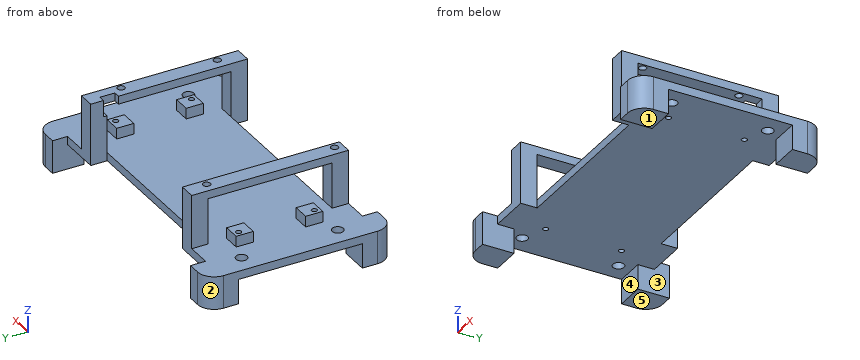
```python
from build123d import *

# Parameters (mm, degrees)
SKETCH1_W             = 112.9284
SKETCH1_H             = 57.214943904
BOSS_EXTRUDE1_DEPTH   = 3.81
BOSS_EXTRUDE2_START   = 11.43
BOSS_EXTRUDE2_DEPTH   = 11.43
CUT_EXTRUDE1_REACH    = 85.521
SKETCH3_R             = 2.58
SKETCH4_W             = 7.786771744
SKETCH4_H             = 7.895685894
BOSS_EXTRUDE3_DEPTH   = 5
CUT_EXTRUDE2_REACH    = 86.577
SKETCH5_R             = 1.25
SKETCH8_W             = 7.62
SKETCH8_H             = 7.62
BOSS_EXTRUDE4_DEPTH   = 24.892
BOSS_EXTRUDE4_2_DEPTH = 24.892
BOSS_EXTRUDE4_3_DEPTH = 24.892
BOSS_EXTRUDE4_4_DEPTH = 24.892
SKETCH9_W             = 7.62
SKETCH9_H             = 7.62
BOSS_EXTRUDE5_DEPTH   = 3.81
BOSS_EXTRUDE6_REACH   = 106.193
SKETCH10_W            = 7.62
SKETCH10_H            = 3.70730408
BOSS_EXTRUDE7_REACH   = 128.11
SKETCH11_W            = 3.81
SKETCH11_H            = 7.62
BOSS_EXTRUDE8_REACH   = 128.11
SKETCH12_W            = 3.81
SKETCH12_H            = 7.62
SKETCH14_R            = 1.7018
CUT_EXTRUDE3_DEPTH    = 3.81
SKETCH16_W            = 2.93944059
SKETCH16_H            = 6.893445181
CUT_EXTRUDE4_DEPTH    = 7.62


with BuildPart() as part:
    # Sketch1 → Boss-Extrude1 (new body)
    with BuildSketch(Plane.XY):
        with BuildLine():
            Line((-56.4642, -28.607471952), (-56.4642, 28.607471952))
            Line((-56.4642, 28.607471952), (-56.4642, 43.18))
            Line((-56.4642, 43.18), (-62.23, 43.18))
            ThreePointArc((-62.23, 43.18), (-67.618153673, 40.948153673), (-69.85, 35.56))
            Line((-69.85, 35.56), (-69.85, -35.56))
            ThreePointArc((-69.85, -35.56), (-67.618153673, -40.948153673), (-62.23, -43.18))
            Line((-62.23, -43.18), (-56.4642, -43.18))
            Line((-56.4642, -43.18), (-56.4642, -28.607471952))
        make_face()
        Rectangle(SKETCH1_W, SKETCH1_H)
        with BuildLine():
            Line((56.4642, 43.18), (56.4642, 28.607471952))
            Line((56.4642, 28.607471952), (56.4642, -28.607471952))
            Line((56.4642, -28.607471952), (56.4642, -43.18))
            Line((56.4642, -43.18), (62.23, -43.18))
            ThreePointArc((62.23, -43.18), (67.618153673, -40.948153673), (69.85, -35.56))
            Line((69.85, -35.56), (69.85, 35.56))
            ThreePointArc((69.85, 35.56), (67.618153673, 40.948153673), (62.23, 43.18))
            Line((62.23, 43.18), (56.4642, 43.18))
        make_face()
    extrude(amount=BOSS_EXTRUDE1_DEPTH)

    # Sketch2 → Boss-Extrude2 (add)
    with BuildSketch(Plane(origin=(0, 0, 0), x_dir=(-1, 0, 0), z_dir=(0, 0, -1)).offset(BOSS_EXTRUDE2_START)):
        with BuildLine():
            Line((-62.23, 43.18), (-56.4642, 43.18))
            Line((-56.4642, 43.18), (-56.4642, 28.607471952))
            Line((-56.4642, 28.607471952), (-69.85, 28.607471952))
            Line((-69.85, 28.607471952), (-69.85, 35.56))
            ThreePointArc((-69.85, 35.56), (-67.618153673, 40.948153673), (-62.23, 43.18))
        make_face()
        with BuildLine():
            Line((69.85, 28.607471952), (56.4642, 28.607471952))
            Line((56.4642, 28.607471952), (56.4642, 43.18))
            Line((56.4642, 43.18), (62.23, 43.18))
            ThreePointArc((62.23, 43.18), (67.618153673, 40.948153673), (69.85, 35.56))
            Line((69.85, 35.56), (69.85, 28.607471952))
        make_face()
        with BuildLine():
            Line((69.85, -35.56), (69.85, -28.607471952))
            Line((69.85, -28.607471952), (56.4642, -28.607471952))
            Line((56.4642, -28.607471952), (56.4642, -43.18))
            Line((56.4642, -43.18), (62.23, -43.18))
            ThreePointArc((62.23, -43.18), (67.618153673, -40.948153673), (69.85, -35.56))
        make_face()
        with BuildLine():
            Line((-69.85, -28.607471952), (-56.4642, -28.607471952))
            Line((-56.4642, -28.607471952), (-56.4642, -43.18))
            Line((-56.4642, -43.18), (-62.23, -43.18))
            ThreePointArc((-62.23, -43.18), (-67.618153673, -40.948153673), (-69.85, -35.56))
            Line((-69.85, -35.56), (-69.85, -28.607471952))
        make_face()
    extrude(amount=-BOSS_EXTRUDE2_DEPTH)

    # Sketch3 → Cut-Extrude1 (cut, up to next)
    with BuildSketch(Plane.XY.offset(3.81), mode=Mode.PRIVATE) as cut_extrude1_sk1:
        with Locations((-61.0842, 22.2292)):
            Circle(SKETCH3_R)
    cut_extrude1_tool1 = extrude(cut_extrude1_sk1.sketch, amount=-CUT_EXTRUDE1_REACH, mode=Mode.PRIVATE) & part.part
    # Sketch3 → Cut-Extrude1 (cut, up to next)
    with BuildSketch(Plane.XY.offset(3.81), mode=Mode.PRIVATE) as cut_extrude1_sk2:
        with Locations((-61.0842, -22.2208)):
            Circle(SKETCH3_R)
    cut_extrude1_tool2 = extrude(cut_extrude1_sk2.sketch, amount=-CUT_EXTRUDE1_REACH, mode=Mode.PRIVATE) & part.part
    # Sketch3 → Cut-Extrude1 (cut, up to next)
    with BuildSketch(Plane.XY.offset(3.81), mode=Mode.PRIVATE) as cut_extrude1_sk3:
        with Locations((61.0958, -22.2208)):
            Circle(SKETCH3_R)
    cut_extrude1_tool3 = extrude(cut_extrude1_sk3.sketch, amount=-CUT_EXTRUDE1_REACH, mode=Mode.PRIVATE) & part.part
    # Sketch3 → Cut-Extrude1 (cut, up to next)
    with BuildSketch(Plane.XY.offset(3.81), mode=Mode.PRIVATE) as cut_extrude1_sk4:
        with Locations((61.0958, 22.2292)):
            Circle(SKETCH3_R)
    cut_extrude1_tool4 = extrude(cut_extrude1_sk4.sketch, amount=-CUT_EXTRUDE1_REACH, mode=Mode.PRIVATE) & part.part
    add(cut_extrude1_tool1.solids().sort_by_distance((-61.0842, 22.2292, 3.81))[0], mode=Mode.SUBTRACT)
    add(cut_extrude1_tool2.solids().sort_by_distance((-61.0842, -22.2208, 3.81))[0], mode=Mode.SUBTRACT)
    add(cut_extrude1_tool3.solids().sort_by_distance((61.0958, -22.2208, 3.81))[0], mode=Mode.SUBTRACT)
    add(cut_extrude1_tool4.solids().sort_by_distance((61.0958, 22.2292, 3.81))[0], mode=Mode.SUBTRACT)

    # Sketch4 → Boss-Extrude3 (add)
    with BuildSketch(Plane.XY.offset(3.81)):
        with Locations((-48.862414128, 16.054657053)):
            Rectangle(SKETCH4_W, SKETCH4_H)
        with Locations((48.862414128, 16.054657053)):
            Rectangle(SKETCH4_W, SKETCH4_H)
        with Locations((48.862414128, -16.054657053)):
            Rectangle(SKETCH4_W, SKETCH4_H)
        with Locations((-48.862414128, -16.054657053)):
            Rectangle(SKETCH4_W, SKETCH4_H)
    extrude(amount=BOSS_EXTRUDE3_DEPTH)

    # Sketch5 → Cut-Extrude2 (cut, up to next)
    with BuildSketch(Plane.XY.offset(8.81), mode=Mode.PRIVATE) as cut_extrude2_sk1:
        with Locations((50.2442, 17.5025)):
            Circle(SKETCH5_R)
    cut_extrude2_tool1 = extrude(cut_extrude2_sk1.sketch, amount=-CUT_EXTRUDE2_REACH, mode=Mode.PRIVATE) & part.part
    # Sketch5 → Cut-Extrude2 (cut, up to next)
    with BuildSketch(Plane.XY.offset(8.81), mode=Mode.PRIVATE) as cut_extrude2_sk2:
        with Locations((50.2442, -17.4975)):
            Circle(SKETCH5_R)
    cut_extrude2_tool2 = extrude(cut_extrude2_sk2.sketch, amount=-CUT_EXTRUDE2_REACH, mode=Mode.PRIVATE) & part.part
    # Sketch5 → Cut-Extrude2 (cut, up to next)
    with BuildSketch(Plane.XY.offset(8.81), mode=Mode.PRIVATE) as cut_extrude2_sk3:
        with Locations((-50.2558, -17.4975)):
            Circle(SKETCH5_R)
    cut_extrude2_tool3 = extrude(cut_extrude2_sk3.sketch, amount=-CUT_EXTRUDE2_REACH, mode=Mode.PRIVATE) & part.part
    # Sketch5 → Cut-Extrude2 (cut, up to next)
    with BuildSketch(Plane.XY.offset(8.81), mode=Mode.PRIVATE) as cut_extrude2_sk4:
        with Locations((-50.2558, 17.5025)):
            Circle(SKETCH5_R)
    cut_extrude2_tool4 = extrude(cut_extrude2_sk4.sketch, amount=-CUT_EXTRUDE2_REACH, mode=Mode.PRIVATE) & part.part
    add(cut_extrude2_tool1.solids().sort_by_distance((50.2442, 17.5025, 8.81))[0], mode=Mode.SUBTRACT)
    add(cut_extrude2_tool2.solids().sort_by_distance((50.2442, -17.4975, 8.81))[0], mode=Mode.SUBTRACT)
    add(cut_extrude2_tool3.solids().sort_by_distance((-50.2558, -17.4975, 8.81))[0], mode=Mode.SUBTRACT)
    add(cut_extrude2_tool4.solids().sort_by_distance((-50.2558, 17.5025, 8.81))[0], mode=Mode.SUBTRACT)



with BuildPart() as body_2:
    # Sketch8 → Boss-Extrude4 (new body)
    with BuildSketch(Plane.XY.offset(3.81)):
        with Locations((-41.297898441, 32.417471952)):
            Rectangle(SKETCH8_W, SKETCH8_H)
    extrude(amount=BOSS_EXTRUDE4_DEPTH)


with BuildPart() as body_3:
    # Sketch8 → Boss-Extrude4 2 (new body)
    with BuildSketch(Plane.XY.offset(3.81)):
        with Locations((41.297898441, 32.417471952)):
            Rectangle(SKETCH8_W, SKETCH8_H)
    extrude(amount=BOSS_EXTRUDE4_2_DEPTH)


with BuildPart() as body_4:
    # Sketch8 → Boss-Extrude4 3 (new body)
    with BuildSketch(Plane.XY.offset(3.81)):
        with Locations((41.297898441, -32.417471952)):
            Rectangle(SKETCH8_W, SKETCH8_H)
    extrude(amount=BOSS_EXTRUDE4_3_DEPTH)


with BuildPart() as body_5:
    # Sketch8 → Boss-Extrude4 4 (new body)
    with BuildSketch(Plane.XY.offset(3.81)):
        with Locations((-41.297898441, -32.417471952)):
            Rectangle(SKETCH8_W, SKETCH8_H)
    extrude(amount=BOSS_EXTRUDE4_4_DEPTH)


with BuildPart() as part_1:
    add(part.part)

    add(body_2.part)  # Boss-Extrude5 merges body 2

    add(body_3.part)  # Boss-Extrude5 merges body 3

    add(body_4.part)  # Boss-Extrude5 merges body 4

    add(body_5.part)  # Boss-Extrude5 merges body 5
    # Sketch9 → Boss-Extrude5 (add)
    with BuildSketch(Plane.XY.offset(3.81)):
        with Locations((41.297898441, 32.417471952)):
            Rectangle(SKETCH9_W, SKETCH9_H)
        with Locations((-41.297898441, 32.417471952)):
            Rectangle(SKETCH9_W, SKETCH9_H)
        with Locations((-41.297898441, -32.417471952)):
            Rectangle(SKETCH9_W, SKETCH9_H)
        with Locations((41.297898441, -32.417471952)):
            Rectangle(SKETCH9_W, SKETCH9_H)
    extrude(amount=-BOSS_EXTRUDE5_DEPTH)

    # Sketch10 → Boss-Extrude6 (add, up to next)
    with BuildSketch(Plane(origin=(0, -28.607471952, 0), x_dir=(1, 0, 0), z_dir=(0, 1, 0)), mode=Mode.PRIVATE) as boss_extrude6_sk1:
        with Locations((-41.297898441, -26.84834796)):
            Rectangle(SKETCH10_W, SKETCH10_H)
    boss_extrude6_tool1 = extrude(boss_extrude6_sk1.sketch, amount=BOSS_EXTRUDE6_REACH, mode=Mode.PRIVATE) - part_1.part
    # Sketch10 → Boss-Extrude6 (add, up to next)
    with BuildSketch(Plane(origin=(0, -28.607471952, 0), x_dir=(1, 0, 0), z_dir=(0, 1, 0)), mode=Mode.PRIVATE) as boss_extrude6_sk2:
        with Locations((41.297898441, -26.84834796)):
            Rectangle(SKETCH10_W, SKETCH10_H)
    boss_extrude6_tool2 = extrude(boss_extrude6_sk2.sketch, amount=BOSS_EXTRUDE6_REACH, mode=Mode.PRIVATE) - part_1.part
    add(boss_extrude6_tool1.solids().sort_by_distance((-41.297898, -28.607472, 26.848348))[0])
    add(boss_extrude6_tool2.solids().sort_by_distance((41.297898, -28.607472, 26.848348))[0])

    # Sketch11 → Boss-Extrude7 (add, up to next)
    with BuildSketch(Plane.ZY.offset(45.107898441), mode=Mode.PRIVATE) as boss_extrude7_sk1:
        with Locations((1.905, -32.417471952)):
            Rectangle(SKETCH11_W, SKETCH11_H)
    boss_extrude7_tool1 = extrude(boss_extrude7_sk1.sketch, amount=BOSS_EXTRUDE7_REACH, mode=Mode.PRIVATE) - part_1.part
    # Sketch11 → Boss-Extrude7 (add, up to next)
    with BuildSketch(Plane.ZY.offset(45.107898441), mode=Mode.PRIVATE) as boss_extrude7_sk2:
        with Locations((1.905, 32.417471952)):
            Rectangle(SKETCH11_W, SKETCH11_H)
    boss_extrude7_tool2 = extrude(boss_extrude7_sk2.sketch, amount=BOSS_EXTRUDE7_REACH, mode=Mode.PRIVATE) - part_1.part
    add(boss_extrude7_tool1.solids().sort_by_distance((-45.107898, -32.417472, 1.905))[0])
    add(boss_extrude7_tool2.solids().sort_by_distance((-45.107898, 32.417472, 1.905))[0])

    # Sketch12 → Boss-Extrude8 (add, up to next)
    with BuildSketch(Plane(origin=(45.107898441, 0, 0), x_dir=(0, 0, -1), z_dir=(1, 0, 0)), mode=Mode.PRIVATE) as boss_extrude8_sk1:
        with Locations((-1.905, 32.417471952)):
            Rectangle(SKETCH12_W, SKETCH12_H)
    boss_extrude8_tool1 = extrude(boss_extrude8_sk1.sketch, amount=BOSS_EXTRUDE8_REACH, mode=Mode.PRIVATE) - part_1.part
    # Sketch12 → Boss-Extrude8 (add, up to next)
    with BuildSketch(Plane(origin=(45.107898441, 0, 0), x_dir=(0, 0, -1), z_dir=(1, 0, 0)), mode=Mode.PRIVATE) as boss_extrude8_sk2:
        with Locations((-1.905, -32.417471952)):
            Rectangle(SKETCH12_W, SKETCH12_H)
    boss_extrude8_tool2 = extrude(boss_extrude8_sk2.sketch, amount=BOSS_EXTRUDE8_REACH, mode=Mode.PRIVATE) - part_1.part
    add(boss_extrude8_tool1.solids().sort_by_distance((45.107898, 32.417472, 1.905))[0])
    add(boss_extrude8_tool2.solids().sort_by_distance((45.107898, -32.417472, 1.905))[0])

    # Sketch14 → Cut-Extrude3 (cut)
    with BuildSketch(Plane.XY.offset(28.702)):
        with Locations((-40.34905784, 26.641762983)):
            Circle(SKETCH14_R)
        with Locations((-40.34905784, -32.445162443)):
            Circle(SKETCH14_R)
        with Locations((42.691835463, 19.276786892)):
            Circle(SKETCH14_R)
        with Locations((42.691835463, -25.172251079)):
            Circle(SKETCH14_R)
    extrude(amount=-CUT_EXTRUDE3_DEPTH, mode=Mode.SUBTRACT)

    # Sketch16 → Cut-Extrude4 (cut)
    with BuildSketch(Plane.XY.offset(28.702)):
        with Locations((38.957618736, 26.875922591)):
            Rectangle(SKETCH16_W, SKETCH16_H)
    extrude(amount=-CUT_EXTRUDE4_DEPTH, mode=Mode.SUBTRACT)


solid = part_1.part
```
Model file for the job. Use its own axes, mm. Face numbers are marked on the shaded views. A direction names the side the tool comes from. Coordinates: 2 decimals unless noted, no trailing zeros. Order: outer loops, then holes, each group sorted by start corner. A loop starts at its lowest first (then second) coordinate and runs counter-clockwise, first axis right, second up. Notation, with made-up numbers: (69, 58.25) - (123, 58.25) arc R12 ccw to (123, 72.25) - close; hole circle Ø3 at (35.5, -39.5). An arc over 180 degrees is marked (long way). Return JSON: item names as keys, results as strings. Group by question number.
1) Mould opens along X. For the marked faces 1, 2 and 3 say: released by +X, released by -X, zero draft, split by the parting line, or undercut.
2) Saw through at A-A, the plane y = -9.5. Write the cut outline in (x, z).
3) Probe line 1 (Y direction, x = 57, z = -8.5); line 2 (Z direction, x = -26, y = -16.5); line 3 (Z direction, x = -61, y = -38.5). List the from-to ranges inside material, lowest first. Write a range as from..to.
4) Flat gauge pins, fed straight in: P1, Ø5.5, axis at x = -43, z = 9, coming from the -Y side; P2, Ø2.5, axis at x = -40, z = 18.5, coming from the +Y side; P3, Ø1.5, axis at x = 50, z = 5.5, coming from the -Y side; P4, Ø12, axis at y = 33, z = 5.5, coming from the +X side. Where does each tip first touch, or does it go through?
5) Saw through at C-C, the plane x = 47. Write the cut outline in (y, z).
6) Saw through at D-D, the plane z = 14.5. Write the cut outline in (x, y).
7) Tool access for the marked faces 4 and 5: list every direction of +Z, -Z, +X, -X, +Y, -Y with a clear straight run to the whole face (end or side of a thin tool).
8) Saw through at B-B, the plane z = -9. Write the cut outline in (x, y), plus the area to 3 significant figures.
Values found:
{
 "1": {"face 1": "zero draft", "face 2": "released by -X", "face 3": "undercut"},
 "2": {"outline": "(-69.85, 0) - (69.85, 0) - (69.85, 3.81) - (-69.85, 3.81) - close; (-45.11, 24.99) - (-37.49, 24.99) - (-37.49, 28.7) - (-45.11, 28.7) - close; (37.49, 24.99) - (45.11, 24.99) - (45.11, 28.7) - (37.49, 28.7) - close"},
 "3": {"line 1": "y = -43.18..-28.61, 28.61..43.18", "line 2": "z = 0..3.81", "line 3": "z = -11.43..3.81"},
 "4": {"P1": "stops at y = -36.23", "P2": "stops at y = 36.23", "P3": "stops at y = -20", "P4": "stops at x = 69.85"},
 "5": {"outline": "(-36.23, 0) - (36.23, 0) - (36.23, 3.81) - (20, 3.81) - (20, 8.81) - (12.11, 8.81) - (12.11, 3.81) - (-12.11, 3.81) - (-12.11, 8.81) - (-20, 8.81) - (-20, 3.81) - (-36.23, 3.81) - close"},
 "6": {"outline": "(-45.11, -36.23) - (-37.49, -36.23) - (-37.49, -28.61) - (-45.11, -28.61) - close; (-45.11, 28.61) - (-37.49, 28.61) - (-37.49, 36.23) - (-45.11, 36.23) - close; (37.49, -36.23) - (45.11, -36.23) - (45.11, -28.61) - (37.49, -28.61) - close; (37.49, 28.61) - (45.11, 28.61) - (45.11, 36.23) - (37.49, 36.23) - close"},
 "7": {"face 4": "-Z, +X, -X", "face 5": "-Z, +X, -X, +Y, -Y"},
 "8": {"outline": "(-69.85, -35.56) arc R7.62 ccw to (-62.23, -43.18) - (-56.46, -43.18) - (-56.46, -28.61) - (-69.85, -28.61) - close; (-69.85, 28.61) - (-56.46, 28.61) - (-56.46, 43.18) - (-62.23, 43.18) arc R7.62 ccw to (-69.85, 35.56) - close; (56.46, -43.18) - (62.23, -43.18) arc R7.62 ccw to (69.85, -35.56) - (69.85, -28.61) - (56.46, -28.61) - close; (56.46, 28.61) - (69.85, 28.61) - (69.85, 35.56) arc R7.62 ccw to (62.23, 43.18) - (56.46, 43.18) - close", "area": "730 mm²"}
}
